The model under review builds one solid part; all positions refer to its coordinate system, in mm. A direction names the side the tool comes from. Round coordinates to 2 decimals unless told otherwise and drop trailing zeros. Order: outer loops, then holes, each group sorted by start corner. A loop starts at its lowest first (then second) coordinate and runs counter-clockwise, first axis right, second up.
from build123d import *

# Parameters (mm, degrees)
SKETCH_1_W      = 10
SKETCH_1_H      = 10
SKETCH_1_W_2    = 180
SKETCH_1_H_2    = 35
EXTRUDE_1_DEPTH = 10
SKETCH_2_W      = 10
SKETCH_2_H      = 10
EXTRUDE_2_DEPTH = 400


with BuildPart() as part:
    # 草图1 → 凸台-拉伸1 (new body)
    with BuildSketch(Plane(origin=(0, 0, 0), x_dir=(1, 0, 0), z_dir=(0, 1, 0))):
        with Locations((-95, 0)):
            Rectangle(SKETCH_1_W, SKETCH_1_H)
        Rectangle(SKETCH_1_W_2, SKETCH_1_H)
        with Locations((-95, -22.5)):
            Rectangle(SKETCH_1_W, SKETCH_1_H_2)
        with Locations((-95, 22.5)):
            Rectangle(SKETCH_1_W, SKETCH_1_H_2)
        with Locations((95, 22.5)):
            Rectangle(SKETCH_1_W, SKETCH_1_H_2)
        with Locations((95, 0)):
            Rectangle(SKETCH_1_W, SKETCH_1_H)
        with Locations((95, -22.5)):
            Rectangle(SKETCH_1_W, SKETCH_1_H_2)
    extrude(amount=EXTRUDE_1_DEPTH)

    # 草图2 → 凸台-拉伸2 (add)
    with BuildSketch(Plane(origin=(0, 10, 0), x_dir=(1, 0, 0), z_dir=(0, 1, 0))):
        with Locations((-95, 0)):
            Rectangle(SKETCH_2_W, SKETCH_2_H)
        with Locations((95, 0)):
            Rectangle(SKETCH_2_W, SKETCH_2_H)
    extrude(amount=EXTRUDE_2_DEPTH)


solid = part.part
(1) To check wall thickness, follow L1, parallel to X at y = 21, z = 2; L2, parallel to Y at x = -86.5, z = -4. State the ranges of each line that lie inside material, in increasing order.
(2) Clearance check with flat-ended pins moving along their axes: P1, Ø3, axis at x = 94, z = 29.5, coming from the +Y side; P2, Ø12, axis at y = 318, z = 11.5, coming from the +X side; P3, Ø4, axis at x = -3, z = -2, coming from the -Y side; P4, Ø5, axis at x = -96, y = 135, coming from the +Z side. State where each tip first meets the part, or that it passes through.
(3) We need section B-B (z = 10.5). Give the boundary of the cut face in (x, y), and give its area (3 significant figures).
(4) Tool access review of faces 1 (the flat face through (-1, 10, 0)), 2 (the flat face through (90, 5, 23)), 3 (the flat face through (90, 5, -22)): name each direction out of +Z, -Z, +X, -X, +Y, -Y from which nothing blocks a thin tool from reaching the whole face with its end or side.
(5) We need section C-C (x = 3). Give the boundary of the cut face in (y, z).
(6) We need section A-A (y = 145). Give the boundary of the cut face in (x, z), and give its area (3 significant figures).
(7) The part is to be moulded in two halves that separate along X. For faces 4 (the flat face through (-95, 5, -40)), 5 (the flat face through (-90, 5, -22)), say which applies: pulls with the +X half, pulls with the -X half, needs draft (parallel to the pull), parting line crosses it, or undercut.
Verdict:
1. L1: x = -100 to -90, 90 to 100
1. L2: y = 0 to 10
2. P1: stops at y = 10
2. P2: passes through
2. P3: stops at y = 0
2. P4: stops at z = 5
3. outline: (-100, 0) - (-90, 0) - (-90, 10) - (-100, 10) - close; (90, 0) - (100, 0) - (100, 10) - (90, 10) - close
3. area: 200 mm2
4. face 1: +Z, -Z, +Y
4. face 2: +Z, +Y, -Y
4. face 3: -Z, +Y, -Y
5. outline: (0, -5) - (10, -5) - (10, 5) - (0, 5) - close
6. outline: (-100, -5) - (-90, -5) - (-90, 5) - (-100, 5) - close; (90, -5) - (100, -5) - (100, 5) - (90, 5) - close
6. area: 200 mm2
7. face 4: needs draft
7. face 5: undercut
